```python
from build123d import *

# Parameters (mm, degrees)
EXTRUDE_WHEEL_DEPTH        = 10
CIRPATTERN1_COUNT          = 26
SKETCH4_R                  = 29
BOSS_EXTRUDE1_DEPTH        = 5
BEARING_HOLE_R             = 5.18
CUT_BEARING_HOLE_DEPTH     = 16
PCB_INSET_CUT_DEPTH        = 1
PCB_INSET_CUT_2_DEPTH      = 1
PCB_OUTPUT_HOLES_R         = 0.6
PCB_OUTPUT_HOLES_CUT_DEPTH = 15
SKETCH5_R                  = 1.5875
ALIGNMENT_PIN_CUTOUT_DEPTH = 15
SKETCH7_R                  = 6.35
CUT_EXTRUDE2_DEPTH         = 9


with BuildPart() as part:
    # Wheel → Extrude wheel (new body)
    with BuildSketch(Plane(origin=(0, 0, 0), x_dir=(1, 0, 0), z_dir=(0, 1, 0))):
        with BuildLine():
            Line((0, 0), (29.128254523, 7.179469929))
            Line((29.128254523, 7.179469929), (30.341931795, 7.478614509))
            ThreePointArc((30.341931795, 7.478614509), (31.616410176, 5.808198613), (31.087663821, 3.774725795))
            ThreePointArc((31.087663821, 3.774725795), (30.249976155, 1.847846509), (31.25, 0))
            Line((31.25, 0), (30, 0))
            Line((30, 0), (0, 0))
        make_face()
    extrude_wheel = extrude(amount=EXTRUDE_WHEEL_DEPTH)

    # CirPattern1: Extrude wheel ×26 about axis
    cirpattern1_axis = Axis((0, 0, 0), (0, 1, 0))
    for i in range(1, CIRPATTERN1_COUNT):
        add(extrude_wheel.rotate(cirpattern1_axis, i * 360 / CIRPATTERN1_COUNT))

    # Sketch4 → Boss-Extrude1 (add)
    with BuildSketch(Plane(origin=(0, 10, 0), x_dir=(1, 0, 0), z_dir=(0, 1, 0))):
        Circle(SKETCH4_R)
    extrude(amount=BOSS_EXTRUDE1_DEPTH)

    # Bearing hole → Cut bearing hole (cut, through all)
    with BuildSketch(Plane(origin=(0, 15, 0), x_dir=(1, 0, 0), z_dir=(0, 1, 0))):
        Circle(BEARING_HOLE_R)
    extrude(amount=-CUT_BEARING_HOLE_DEPTH, mode=Mode.SUBTRACT)

    # PCB inset → PCB inset cut (cut)
    with BuildSketch(Plane(origin=(0, 15, 0), x_dir=(1, 0, 0), z_dir=(0, 1, 0))):
        with BuildLine():
            Line((-1, 27.481812167), (-1, 29.481812167))
            Line((-1, 29.481812167), (1, 29.481812167))
            Line((1, 29.481812167), (1, 27.481812167))
            ThreePointArc((1, 27.481812167), (0, -27.5), (-1, 27.481812167))
        make_face()
    extrude(amount=-PCB_INSET_CUT_DEPTH, mode=Mode.SUBTRACT)

    # PCB inset 2 → PCB inset cut 2 (cut)
    with BuildSketch(Plane.XZ):
        with BuildLine():
            Line((1, -27.481812167), (1, -29.481812167))
            Line((1, -29.481812167), (-1, -29.481812167))
            Line((-1, -29.481812167), (-1, -27.481812167))
            ThreePointArc((-1, -27.481812167), (0, 27.5), (1, -27.481812167))
        make_face()
    extrude(amount=-PCB_INSET_CUT_2_DEPTH, mode=Mode.SUBTRACT)

    # PCB output holes → PCB output holes cut (cut, through all)
    with BuildSketch(Plane(origin=(0, 14, 0), x_dir=(1, 0, 0), z_dir=(0, 1, 0))):
        with Locations((15, 0)):
            Circle(PCB_OUTPUT_HOLES_R)
        with Locations((14.564127261, -3.589734964)):
            Circle(PCB_OUTPUT_HOLES_R)
        with Locations((13.281840385, -6.970847581)):
            Circle(PCB_OUTPUT_HOLES_R)
        with Locations((11.227661223, -9.946839874)):
            Circle(PCB_OUTPUT_HOLES_R)
        with Locations((8.520971201, -12.344757988)):
            Circle(PCB_OUTPUT_HOLES_R)
        with Locations((5.319073306, -14.02524364)):
            Circle(PCB_OUTPUT_HOLES_R)
        with Locations((1.808050204, -14.890633111)):
            Circle(PCB_OUTPUT_HOLES_R)
        with Locations((-1.808050204, -14.890633111)):
            Circle(PCB_OUTPUT_HOLES_R)
        with Locations((-5.319073306, -14.02524364)):
            Circle(PCB_OUTPUT_HOLES_R)
        with Locations((-8.520971201, -12.344757988)):
            Circle(PCB_OUTPUT_HOLES_R)
        with Locations((-11.227661223, -9.946839874)):
            Circle(PCB_OUTPUT_HOLES_R)
        with Locations((-13.281840385, -6.970847581)):
            Circle(PCB_OUTPUT_HOLES_R)
        with Locations((-14.564127261, -3.589734964)):
            Circle(PCB_OUTPUT_HOLES_R)
        with Locations((-15, 0)):
            Circle(PCB_OUTPUT_HOLES_R)
        with Locations((-14.564127261, 3.589734964)):
            Circle(PCB_OUTPUT_HOLES_R)
        with Locations((-13.281840385, 6.970847581)):
            Circle(PCB_OUTPUT_HOLES_R)
        with Locations((-11.227661223, 9.946839874)):
            Circle(PCB_OUTPUT_HOLES_R)
        with Locations((-8.520971201, 12.344757988)):
            Circle(PCB_OUTPUT_HOLES_R)
        with Locations((-5.319073306, 14.02524364)):
            Circle(PCB_OUTPUT_HOLES_R)
        with Locations((-1.808050204, 14.890633111)):
            Circle(PCB_OUTPUT_HOLES_R)
        with Locations((1.808050204, 14.890633111)):
            Circle(PCB_OUTPUT_HOLES_R)
        with Locations((5.319073306, 14.02524364)):
            Circle(PCB_OUTPUT_HOLES_R)
        with Locations((8.520971201, 12.344757988)):
            Circle(PCB_OUTPUT_HOLES_R)
        with Locations((11.227661223, 9.946839874)):
            Circle(PCB_OUTPUT_HOLES_R)
        with Locations((13.281840385, 6.970847581)):
            Circle(PCB_OUTPUT_HOLES_R)
        with Locations((14.564127261, 3.589734964)):
            Circle(PCB_OUTPUT_HOLES_R)
    extrude(amount=-PCB_OUTPUT_HOLES_CUT_DEPTH, mode=Mode.SUBTRACT)

    # Sketch5 → Alignment pin cutout (cut, through all)
    with BuildSketch(Plane.XZ.offset(-1)):
        with Locations((0, -25)):
            Circle(SKETCH5_R)
        with Locations((-21.650635095, 12.5)):
            Circle(SKETCH5_R)
        with Locations((21.650635095, 12.5)):
            Circle(SKETCH5_R)
    extrude(amount=-ALIGNMENT_PIN_CUTOUT_DEPTH, mode=Mode.SUBTRACT)

    # Sketch7 → Cut-Extrude2 (cut)
    with BuildSketch(Plane.XZ.offset(-1)):
        Circle(SKETCH7_R)
    extrude(amount=-CUT_EXTRUDE2_DEPTH, mode=Mode.SUBTRACT)


solid = part.part
```
Geometry: final body of the model. Coordinates: model frame, mm. A direction names the side the tool comes from. Round coordinates to 2 decimals unless told otherwise and drop trailing zeros. Loops run counter-clockwise (first coordinate to the right, second up) from the corner with the lowest first, then second, coordinate; pieces in that order, holes last. Notation, with made-up numbers: (-24, -33) -> (22, -33) arc R21 ccw to (22, -4) -> close; hole circle Ø2 at (21, 62). An arc over 180 degrees is marked (long way). Use one line per item in the form item = value. Start each with the question number.
1) Draft query along X for faces 3 (the cylindrical face through (-1.782, 4.93, 30.255)), 4 (the cylindrical face through (-27.532, 4.93, -16.592)), 5 (the cylindrical face through (30.25, 4.93, -1.88)). Return one class per face: released by +X, released by -X, zero draft, split by the parting line, or undercut.
2) Section B-B on y = 7.25. Give the number of separate pieces and of enclosed holes in the cut face, then the cut area to 3 significant figures.
3) First-contact query: P1, Ø1.4, axis at x = 5.32, z = 14.03, coming from the -Y side; P2, Ø1.9, axis at x = -21.65, z = 12.5, coming from the -Y side; P3, Ø6, axis at x = -18.5, y = 11.5, coming from the -Z side; P4, Ø8, axis at y = 5.5, z = -24.5, coming from the +X side. Flat tips, straight axial feed; report the tip coordinate or a pass-through.
4) Section A-A on x = -24.5. Output: boundary loops of the cut face in (y, z).
5) Access query for faces 1 (the flat face through (6, 14, -1)), 2 (the cylindrical face through (-25.91, 4.93, 15.72)). Directions: +Z, -Z, +X, -X, +Y, -Y. A direction counts if a zero-diameter tool reaches every point of the face in a straight line with its end or side. Return the directions, or none.
6) Line query: L1, parallel to X at y = 11.25, z = -12; L2, parallel to Z at x = 15, y = 6.5; L3, parallel to Z at x = -9, y = 2.25. Output: solid intervals per line, ascending.
Response:
q1.face_3 = undercut
q1.face_4 = released by -X
q1.face_5 = released by +X
q2.separate_pieces = 1
q2.enclosed_holes = 30
q2.area = 2,890 mm^2
q3.P1 = 1
q3.P2 = through
q3.P3 = -27.81
q3.P4 = 24.44
q4.outline = (0, -18.13) -> (10, -18.13) -> (10, -15.52) -> (15, -15.52) -> (15, -12.49) -> (14, -12.49) -> (14, 12.49) -> (15, 12.49) -> (15, 15.52) -> (10, 15.52) -> (10, 20.47) -> (0, 20.47) -> (0, 12.49) -> (1, 12.49) -> (1, -12.49) -> (0, -12.49) -> close
q5.face_1 = +Y
q5.face_2 = -X, +Y, -Y
q6.L1 = -26.4 to -9.01, -8.03 to 8.03, 9.01 to 26.4
q6.L2 = -26.56 to -4, -3.18 to -0.6, 0.6 to 3.18, 4 to 27.84
q6.L3 = -30.8 to -12.71, -11.98 to 11.98, 12.71 to 28.94
